Work out the finished part from the listing and answer in its coordinate system (mm). A direction names the side the tool comes from. Coordinates: 2 decimals unless noted, no trailing zeros. Order: outer loops, then holes, each group sorted by start corner. A loop starts at its lowest first (then second) coordinate and runs counter-clockwise, first axis right, second up.
1. The part is cut by section B-B, the plane x = 1.67. Give the vertices of the cut face in (y, z).
2. The part is cut by section D-D, the plane x = -5. Give the vertices of the cut face in (y, z).
3. Flat-ended cylindrical pins translate along their axes: pin 1 Ø0.9 at (x, y) = (-1.5, 2) entering from +Z; pin 2 Ø2 at (y, z) = (-0.5, -1.5) entering from -X; pin 3 Ø2 at (x, y) = (-1.5, -1.5) entering from -Z. Find the tip coordinate at first contact, or state that the pin passes through.
4. A tool of negligible diameter and unlimited length cuts with its end or side. For faces 1 (the flat face through (2, 1.6, -7)), 2 (the flat face through (2.6, -1, -8)), 3 (the flat face through (13, -1, -8)), 4 (the flat face through (8, -1, -11.4)), 5 (the flat face through (-5, -0.8, -7)), from which of +Z, -Z, +X, -X, +Y, -Y can it reach the whole face along a straight path? Write none if from no direction.
5. The part is cut by section A-A, the plane y = 0.9. Give the vertices of the cut face in (x, z).
6. Find the intervals of material crossed by probe 1 along X at (y, z) = (0.4, -0.75); probe 2 along Y at (x, z) = (7.5, -5.25); probe 3 along Y at (x, z) = (3.25, -2), in increasing order.
7. The part is cut by section C-C, the plane z = -0.75. Give the vertices of the cut face in (x, y), then the cut area to 4 significant figures.
8. Determine the mould class of faces 6 (the flat face through (8, -1, -4.2)), 7 (the flat face through (8, -2.7, -8)), 8 (the cylindrical face through (4.63, 0.76, -0.48)) for opening direction Z: +Z half, -Z half, draft (parallel to the pull), parting line (faces both ways), or undercut.
```python
from build123d import *

# Parameters (mm, degrees)
SKETCH1_W           = 13.5
SKETCH1_H           = 13.5
BOSS_EXTRUDE1_DEPTH = 1.5
SKETCH2_R           = 0.5
CUT_EXTRUDE1_DEPTH  = 1.5
SKETCH3_R           = 4.8
BOSS_EXTRUDE2_DEPTH = 0.8
SKETCH4_R           = 4.8
BOSS_EXTRUDE3_DEPTH = 2.2
FILLET1_R           = 0.5
SKETCH5_W           = 10.4
SKETCH5_H           = 7.2
BOSS_EXTRUDE4_DEPTH = 2.7
SKETCH7_W           = 1.5
SKETCH7_H           = 0.1
SKETCH8_W           = 4
SKETCH8_H           = 0.1
BOSS_EXTRUDE5_DEPTH = 4


with BuildPart() as part:
    # Sketch1 → Boss-Extrude1 (new body)
    with BuildSketch(Plane(origin=(0, 0, 0), x_dir=(1, 0, 0), z_dir=(0, 1, 0))):
        with Locations((6.75, 6.75)):
            Rectangle(SKETCH1_W, SKETCH1_H)
    extrude(amount=BOSS_EXTRUDE1_DEPTH)

    # Sketch2 → Cut-Extrude1 (cut)
    with BuildSketch(Plane(origin=(0, 1.5, 0), x_dir=(1, 0, 0), z_dir=(0, 1, 0))):
        with Locations(Location((11.83, 0.75, 0), (0, 0, 270))):
            Circle(SKETCH2_R)
        with Locations(Location((9.29, 0.75, 0), (0, 0, 270))):
            Circle(SKETCH2_R)
        with Locations(Location((6.75, 0.75, 0), (0, 0, 270))):
            Circle(SKETCH2_R)
        with Locations(Location((4.21, 0.75, 0), (0, 0, 270))):
            Circle(SKETCH2_R)
        with Locations(Location((1.67, 0.75, 0), (0, 0, 270))):
            Circle(SKETCH2_R)
    extrude(amount=-CUT_EXTRUDE1_DEPTH, mode=Mode.SUBTRACT)

    # Sketch5 → Boss-Extrude4 (add)
    with BuildSketch(Plane.XZ):
        with Locations((7.8, -7.8)):
            Rectangle(SKETCH5_W, SKETCH5_H)
    extrude(amount=BOSS_EXTRUDE4_DEPTH)



with BuildPart() as body_2:
    # Sketch3 → Boss-Extrude2 (new body)
    with BuildSketch(Plane(origin=(0, 0, 0), x_dir=(1, 0, 0), z_dir=(0, 1, 0))):
        with Locations(Location((-5, 6.75, 0), (0, 0, 270))):
            Circle(SKETCH3_R)
    extrude(amount=-BOSS_EXTRUDE2_DEPTH)

    # Sketch4 → Boss-Extrude3 (add)
    with BuildSketch(Plane(origin=(0, 0, 0), x_dir=(1, 0, 0), z_dir=(0, 1, 0))):
        with Locations(Location((-5, 6.75, 0), (0, 0, 270))):
            Circle(SKETCH4_R)
    extrude(amount=BOSS_EXTRUDE3_DEPTH)

    # Fillet1
    fillet1_edges = [body_2.edges().sort_by_distance(p)[0] for p in [
        (-5, -0.8, -11.55),
        (-5, 2.2, -11.55),
    ]]
    fillet(fillet1_edges, radius=FILLET1_R)


with BuildPart() as part_1:
    add(part.part)

    add(body_2.part)  # Sweep1 merges body 2
    # Sweep1: sweep along a path in Sketch6
    with BuildLine(Plane.XY.offset(-6.75)) as sweep1_path:
        Line((-3, 2.2), (-0.684692448, 2.2))
        ThreePointArc((-0.684692448, 2.2), (-0.302009016, 2.123879533), (0.022414333, 1.907106781))
        Line((0.022414333, 1.907106781), (0.136627895, 1.792893219))
        ThreePointArc((0.136627895, 1.792893219), (0.461051244, 1.576120467), (0.843734676, 1.5))
        Line((0.843734676, 1.5), (2.429521114, 1.5))
    # Sketch7 → Sweep1 (sweep)
    with BuildSketch(Plane(origin=(-3, 0, 0), x_dir=(0, 0, -1), z_dir=(1, 0, 0))):
        with Locations((6.75, 2.25)):
            Rectangle(SKETCH7_W, SKETCH7_H)
    sweep(path=sweep1_path.line)

    # Sketch8 → Boss-Extrude5 (add)
    with BuildSketch(Plane(origin=(-3, 0, 0), x_dir=(0, 0, -1), z_dir=(1, 0, 0))):
        with Locations((6.75, 2.25)):
            Rectangle(SKETCH8_W, SKETCH8_H)
    extrude(amount=-BOSS_EXTRUDE5_DEPTH)


solid = part_1.part
```
Geometry says:
1. outline: (0, -13.5) - (1.5, -13.5) - (1.5, -7.5) - (1.6, -7.5) - (1.6, -6) - (1.5, -6) - (1.5, -1.25) - (0, -1.25) - close; (0, -0.25) - (1.5, -0.25) - (1.5, 0) - (0, 0) - close
2. outline: (-0.8, -11.05) arc R0.5 ccw to (-0.3, -11.55) - (1.7, -11.55) arc R0.5 ccw to (2.2, -11.05) - (2.2, -8.75) - (2.3, -8.75) - (2.3, -4.75) - (2.2, -4.75) - (2.2, -2.45) arc R0.5 ccw to (1.7, -1.95) - (-0.3, -1.95) arc R0.5 ccw to (-0.8, -2.45) - close
3. pin 1: stops at z = -3.09
3. pin 2: stops at x = -7.2
3. pin 3: stops at z = -10.33
4. face 1: +Z, -Z, +X, +Y
4. face 2: +Z, -Z, -Y
4. face 3: +Z, -Z, +X, -Y
4. face 4: -Z, +X, -Y
4. face 5: +Z, -Z, -X, -Y
5. outline: circle Ø9.6 at (-5, -6.75); (0, -13.5) - (13.5, -13.5) - (13.5, 0) - (0, 0) - close; hole circle Ø1 at (1.67, -0.75); hole circle Ø1 at (4.21, -0.75); hole circle Ø1 at (6.75, -0.75); hole circle Ø1 at (9.29, -0.75); hole circle Ø1 at (11.83, -0.75)
6. probe 1: x = 0 to 1.17, 2.17 to 3.71, 4.71 to 6.25, 7.25 to 8.79, 9.79 to 11.33, 12.33 to 13.5
6. probe 2: y = -2.7 to 1.5
6. probe 3: y = 0 to 1.5
7. outline: (0, 0) - (1.17, 0) - (1.17, 1.5) - (0, 1.5) - close; (2.17, 0) - (3.71, 0) - (3.71, 1.5) - (2.17, 1.5) - close; (4.71, 0) - (6.25, 0) - (6.25, 1.5) - (4.71, 1.5) - close; (7.25, 0) - (8.79, 0) - (8.79, 1.5) - (7.25, 1.5) - close; (9.79, 0) - (11.33, 0) - (11.33, 1.5) - (9.79, 1.5) - close; (12.33, 0) - (13.5, 0) - (13.5, 1.5) - (12.33, 1.5) - close
7. area: 12.75 mm2
8. face 6: +Z half
8. face 7: draft
8. face 8: undercut
